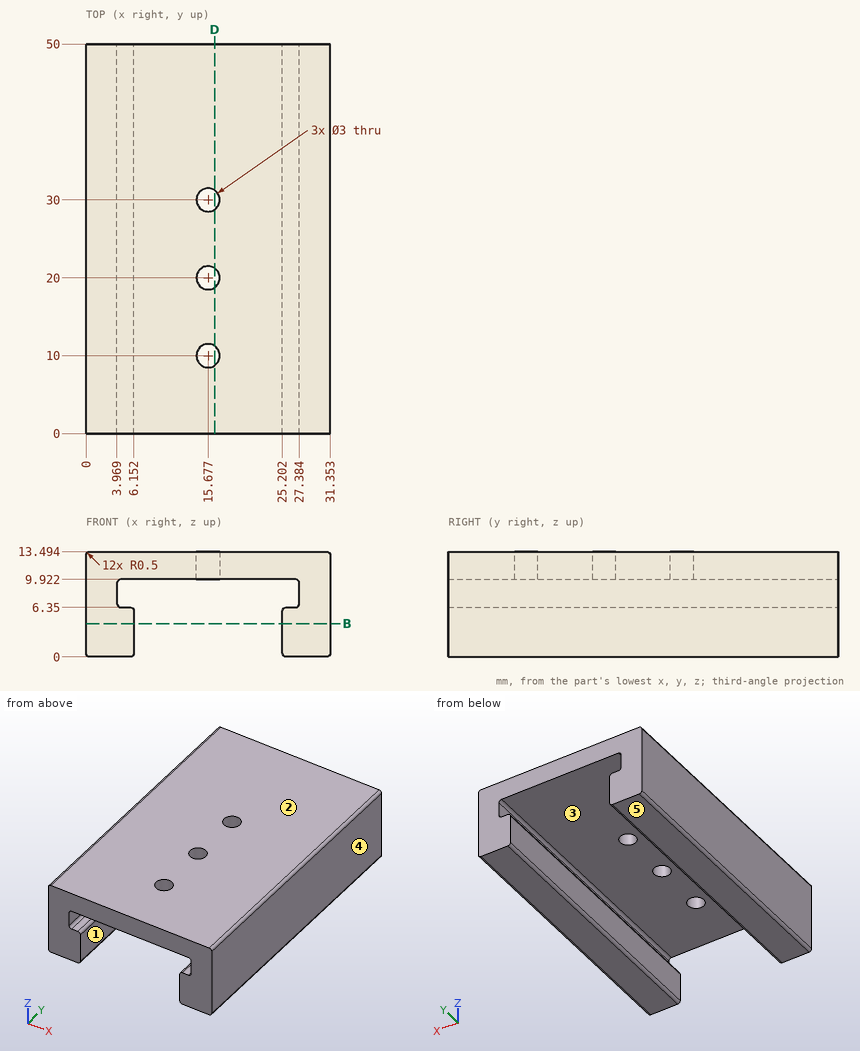
Design review of the part shown in the three views and the two pictorial views. Dimensions are in mm from the part's minimum x, y and z. A direction names the side the tool comes from. Round coordinates to 2 decimals unless told otherwise and drop trailing zeros. Loops run counter-clockwise (first coordinate to the right, second up) from the corner with the lowest first, then second, coordinate; pieces in that order, holes last. Notation, with made-up numbers: M 24,28 L 40,28 A15 ccw 40,41 Z; hole C -37.5,4 d3. An arc over 180 degrees is marked long. Answer as a JSON object with one key per item and string values.
Item 1: We need section D-D, the plane x = 16.5. State the section outline as (y, z) points, and give its area (3 significant figures).
Check sheet entries:
{"outline": "M 0,9.92 L 8.75,9.92 L 8.75,13.49 L 0,13.49 Z; M 11.25,9.92 L 18.75,9.92 L 18.75,13.49 L 11.25,13.49 Z; M 21.25,9.92 L 28.75,9.92 L 28.75,13.49 L 21.25,13.49 Z; M 31.25,9.92 L 50,9.92 L 50,13.49 L 31.25,13.49 Z", "area": "152 mm2"}
Item 2: For line 1 along Z through (x, y) = (5, 23); line 2 along X through (y, z) = (20.5, 9) (1 decimal); line 3 along X through (y, z) = (18, 3), list the stretches that pass through material, from the lowest coordinate up.
Check sheet entries:
{"line 1": "0 to 6.35, 9.92 to 13.49", "line 2": "0 to 4, 27.4 to 31.4", "line 3": "0 to 6.15, 25.2 to 31.35"}
Item 3: Tool access review of the marked faces 1 and 2: name each direction out of +Z, -Z, +X, -X, +Y, -Y from which nothing blocks a thin tool from reaching the whole face with its end or side.
Check sheet entries:
{"face 1": "-Z, +Y, -Y", "face 2": "+Z, +X, -X, +Y, -Y"}
Item 4: We need section B-B, the plane z = 4.25. State the section outline as (x, y) points, and give its area (3 significant figures).
Check sheet entries:
{"outline": "M 0,0 L 6.15,0 L 6.15,50 L 0,50 Z; M 25.2,0 L 31.35,0 L 31.35,50 L 25.2,50 Z", "area": "615 mm2"}
Item 5: Clearance check with flat-ended pins moving along their axes: P1, Ø4, axis at x = 15.68, y = 10, coming from the -Z side; P2, Ø1.8, axis at x = 15.68, y = 20, coming from the -Z side. State where each tip first meets the part, or that it passes through.
Check sheet entries:
{"P1": "z = 9.92", "P2": "through"}
Item 6: The part is to be moulded in two halves that separate along X. For the marked faces 3, 4 and 5, say which applies: +X half, -X half, draft (parallel to the pull), parting line (faces both ways), or undercut.
Check sheet entries:
{"face 3": "undercut", "face 4": "+X half", "face 5": "draft"}
